Can you work these out from the drawing? Everything is in mm from the part's minimum corner. Give positions to 0.01 mm unless a question says otherwise; leave off trailing zeros. Order: outer loops, then holes, each group sorted by start corner. A loop starts at its lowest first (then second) coordinate and runs counter-clockwise, first axis right, second up. Notation, with made-up numbers: (-33, 5) -> (2, 5) arc R15 ccw to (2, 26) -> close; hole circle Ø10 at (64.25, 31.5). An arc over 180 degrees is marked (long way). One line per item, written item: value.
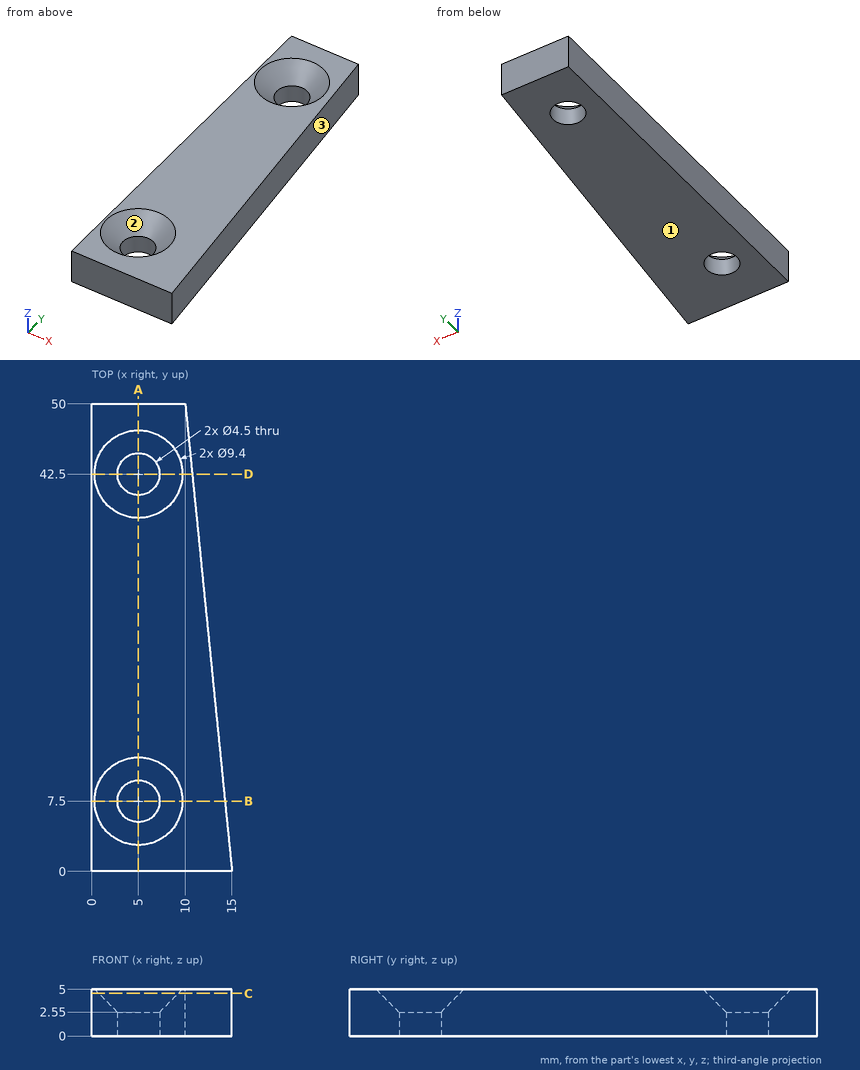
1) For P1, Ø7, axis at x = 5, y = 7.5, coming from the +Z side; P2, Ø6, axis at x = 5, y = 42.5, coming from the +Z side; P3, Ø1.5, axis at y = 27, z = 2, coming from the +X side (3 decimals), each with a flat end and sliding along its axis, tell me the tip position at first contact or that it passes through.
Answer below:
P1: stops at z = 3.8
P2: stops at z = 3.3
P3: stops at x = 12.375
2) Suppose I cut it at C-C, the plane z = 4.55. Write out the boundary of the cut face in (x, y), then the cut area to 3 significant figures.
Answer below:
outline: (0, 0) -> (15, 0) -> (10, 50) -> (0, 50) -> close; hole circle Ø8.5 at (5, 7.5); hole circle Ø8.5 at (5, 42.5)
area: 512 mm2
3) If I drill on line 1 along Y through (x, z) = (5, 2); line 2 along Y through (x, z) = (4.25, 2.75); line 3 along X through (y, z) = (42.5, 1.15), over which ranges is the centre line in solid material (lowest first)?
Answer below:
line 1: y = 0 to 5.25, 9.75 to 40.25, 44.75 to 50
line 2: y = 0 to 5.17, 9.83 to 40.17, 44.83 to 50
line 3: x = 0 to 2.75, 7.25 to 10.75
4) We'd pull the mould along Y, two halves only. Please class the marked faces 1, 2 and 3: +Y half, -Y half, draft (parallel to the pull), parting line (faces both ways), or undercut.
Answer below:
face 1: draft
face 2: undercut
face 3: +Y half
5) Suppose I cut it at D-D, the plane y = 42.5. Write out the boundary of the cut face in (x, z), then the cut area to 3 significant figures.
Answer below:
outline: (0, 0) -> (2.75, 0) -> (2.75, 2.55) -> (0.3, 5) -> (0, 5) -> close; (7.25, 0) -> (10.75, 0) -> (10.75, 5) -> (9.7, 5) -> (7.25, 2.55) -> close
area: 25.2 mm2
6) Suppose I cut it at B-B, the plane y = 7.5. Write out the boundary of the cut face in (x, z).
Answer below:
outline: (0, 0) -> (2.75, 0) -> (2.75, 2.55) -> (0.3, 5) -> (0, 5) -> close; (7.25, 0) -> (14.25, 0) -> (14.25, 5) -> (9.7, 5) -> (7.25, 2.55) -> close
7) Suppose I cut it at A-A, the plane x = 5. Write out the boundary of the cut face in (y, z).
Answer below:
outline: (0, 0) -> (5.25, 0) -> (5.25, 2.55) -> (2.8, 5) -> (0, 5) -> close; (9.75, 0) -> (40.25, 0) -> (40.25, 2.55) -> (37.8, 5) -> (12.2, 5) -> (9.75, 2.55) -> close; (44.75, 0) -> (50, 0) -> (50, 5) -> (47.2, 5) -> (44.75, 2.55) -> close
